Source: three-view drawing plus pictorial views. Frame: mm from the lowest corner of the part. A direction names the side the tool comes from. Give positions to 0.01 mm unless a question says otherwise; leave off trailing zeros. Loops run counter-clockwise (first coordinate to the right, second up) from the corner with the lowest first, then second, coordinate; pieces in that order, holes last. Notation, with made-up numbers: M -24.75,56 L 4.25,56 A20 cw 4.25,89 Z; hole C -31,74 d6. An arc over 180 degrees is marked long. Answer as a JSON object with one key per item and string values. Group by question number.
1) Section query B-B on y = 13.5. Return loops of the section in (x, z), plus the area to 4 significant figures.
2) Section query C-C on x = 60.5. Return loops of the section in (y, z) (1 decimal).
3) Section query A-A on z = 63.5. Return loops of the section in (x, y).
4) Access query for the marked faces 4, 5 and 6. Directions: +Z, -Z, +X, -X, +Y, -Y. A direction counts if a zero-diameter tool reaches every point of the face in a straight line with its end or side. Return the directions, or none.
5) First-contact query: P1, Ø2, axis at x = 24, z = 60.5, coming from the +Y side; P2, Ø21, axis at x = 28, z = 48.5, coming from the -Y side; P3, Ø8.5, axis at x = 59.68, z = 20.75, coming from the -Y side. Flat tips, straight axial feed; report the tip coordinate or a pass-through.
6) Section query D-D on z = 49.25. Count the separate pieces of the cut face and the enclosed holes in it, plus the area to 3 significant figures.
7) Draft query along Z for the marked faces 1, 2 and 3. Return one class per face: +Z half, -Z half, draft (parallel to the pull), parting line (faces both ways), or undercut.
8) Ray query, L1, parallel to Z at x = 35, y = 12.1; L2, parallel to Y at x = 30.5, z = 66.5; L3, parallel to Z at x = 30, y = 15.75 (1 decimal). Return the intervals inside material, ascending.
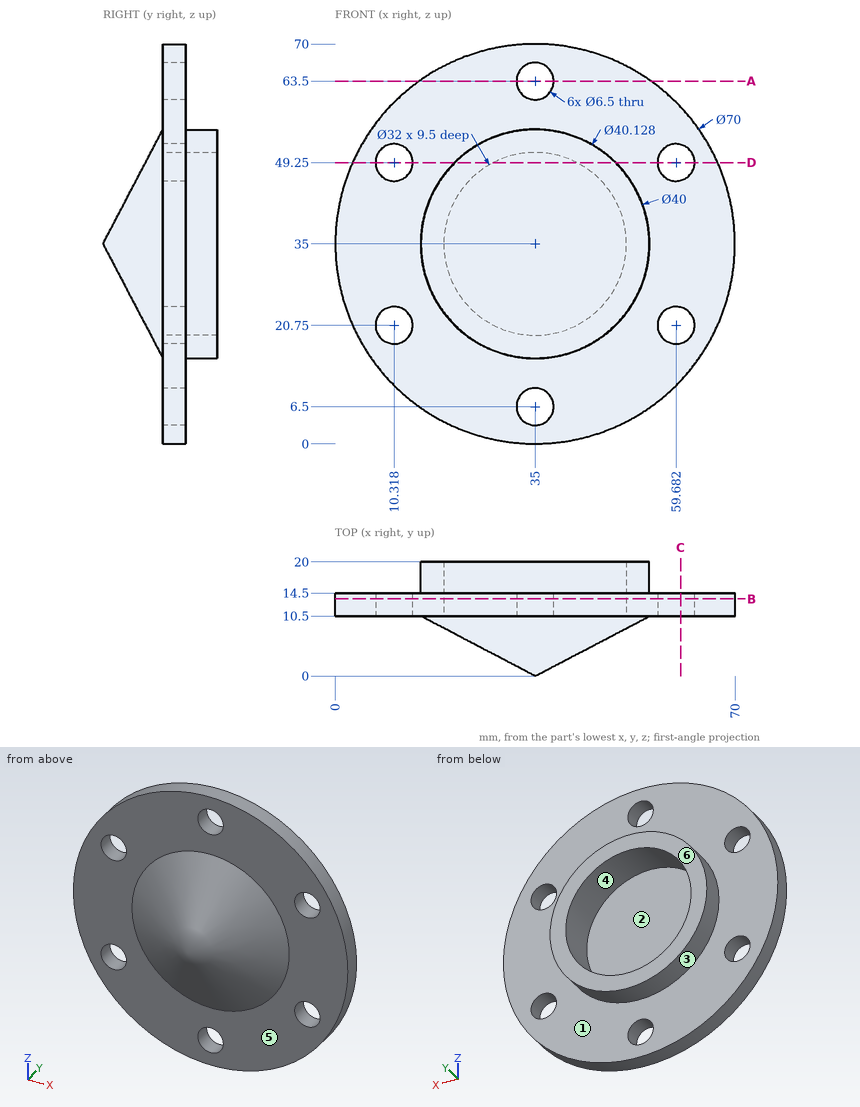
Output:
{
 "1": {"outline": "C 35,35 d70; hole C 10.32,20.75 d6.5; hole C 10.32,49.25 d6.5; hole C 35,35 d32; hole C 35,6.5 d6.5; hole C 35,63.5 d6.5; hole C 59.68,20.75 d6.5; hole C 59.68,49.25 d6.5", "area": "2,845 mm^2"},
 "2": {"outline": "M 10.5,11 L 14.5,11 L 14.5,17.6 L 10.5,17.6 Z; M 10.5,23.9 L 14.5,23.9 L 14.5,46.1 L 10.5,46.1 Z; M 10.5,52.4 L 14.5,52.4 L 14.5,59 L 10.5,59 Z"},
 "3": {"outline": "M 14.68,10.5 L 31.75,10.5 L 31.75,14.5 L 14.68,14.5 Z; M 38.25,10.5 L 55.32,10.5 L 55.32,14.5 L 38.25,14.5 Z"},
 "4": {"face 4": "+Y", "face 5": "-Y", "face 6": "+Z, -Z, +X, -X, +Y"},
 "5": {"P1": "stops at y = 14.5", "P2": "stops at y = 2.46", "P3": "stops at y = 10.5"},
 "6": {"separate pieces": "3", "enclosed holes": "0", "area": "275 mm^2"},
 "7": {"face 1": "draft", "face 2": "undercut", "face 3": "parting line"},
 "8": {"L1": "z = 0 to 3.25, 9.75 to 19, 51 to 60.25, 66.75 to 70", "L2": "y = 10.5 to 14.5", "L3": "z = 15.6 to 19.8, 50.2 to 54.4"}
}
